from build123d import *

# Parameters (mm, degrees)
SKETCH1_R           = 2.286
BOSS_EXTRUDE1_DEPTH = 1.5875
SKETCH2_R           = 2.286
CUT_EXTRUDE1_DEPTH  = 118.348360795
SKETCH3_R           = 1.27
CUT_EXTRUDE2_DEPTH  = 118.348360795
SKETCH4_W           = 2.54
SKETCH4_H           = 6.9596
BOSS_EXTRUDE2_DEPTH = 8.89
CHAMFER1_SIZE       = 1.27
SKETCH5_W           = 10.16
SKETCH5_H           = 2.54
CUT_EXTRUDE3_DEPTH  = 118.673912678
SKETCH6_R           = 1.27
CUT_EXTRUDE4_DEPTH  = 8.89


with BuildPart() as part:
    # Sketch1 → Boss-Extrude1 (new body)
    with BuildSketch(Plane(origin=(0, 0, 0), x_dir=(1, 0, 0), z_dir=(0, 1, 0))):
        Polygon((-25.4, 86.995), (-63.43142, 86.995), (-63.43142, 60.96), (-78.74, 60.96), (-78.74, 25.4), (-71.12, 25.4), (-71.12, -25.4), (-78.74, -25.4), (-78.74, -60.96), (-63.43142, -60.96), (-63.43142, -86.995), (-25.4, -86.995), (-25.4, -79.375), (25.4, -79.375), (25.4, -86.995), (63.43142, -86.995), (63.43142, -60.96), (78.74, -60.96), (78.74, -25.4), (71.12, -25.4), (71.12, 25.4), (78.74, 25.4), (78.74, 60.96), (63.43142, 60.96), (63.43142, 86.995), (25.4, 86.995), (25.4, 79.375), (-25.4, 79.375), align=None)
        with Locations(Location((-57.15, 76.2, 0), (0, 0, 270))):
            Circle(SKETCH1_R, mode=Mode.SUBTRACT)
        with Locations(Location((57.15, 76.2, 0), (0, 0, 270))):
            Circle(SKETCH1_R, mode=Mode.SUBTRACT)
        with Locations(Location((57.15, -76.2, 0), (0, 0, 270))):
            Circle(SKETCH1_R, mode=Mode.SUBTRACT)
        with Locations(Location((-57.15, -76.2, 0), (0, 0, 270))):
            Circle(SKETCH1_R, mode=Mode.SUBTRACT)
    extrude(amount=BOSS_EXTRUDE1_DEPTH)

    # Sketch2 → Cut-Extrude1 (cut, through all)
    with BuildSketch(Plane(origin=(0, 1.5875, 0), x_dir=(1, 0, 0), z_dir=(0, 1, 0))):
        with Locations(Location((-73.66, -30.48, 0), (0, 0, 270))):
            Circle(SKETCH2_R)
        with Locations(Location((-73.66, -55.88, 0), (0, 0, 270))):
            Circle(SKETCH2_R)
        with Locations(Location((73.66, -55.88, 0), (0, 0, 90))):
            Circle(SKETCH2_R)
        with Locations(Location((73.66, -30.48, 0), (0, 0, 90))):
            Circle(SKETCH2_R)
        with Locations(Location((73.66, 30.48, 0), (0, 0, 270))):
            Circle(SKETCH2_R)
        with Locations(Location((73.66, 55.88, 0), (0, 0, 270))):
            Circle(SKETCH2_R)
        with Locations(Location((-73.66, 55.88, 0), (0, 0, 90))):
            Circle(SKETCH2_R)
        with Locations(Location((-73.66, 30.48, 0), (0, 0, 90))):
            Circle(SKETCH2_R)
    extrude(amount=-CUT_EXTRUDE1_DEPTH, mode=Mode.SUBTRACT)

    # Sketch3 → Cut-Extrude2 (cut, through all)
    with BuildSketch(Plane(origin=(0, 1.5875, 0), x_dir=(1, 0, 0), z_dir=(0, 1, 0))):
        with Locations(Location((-50.73142, 66.675, 0), (0, 0, 270))):
            Circle(SKETCH3_R)
        with Locations(Location((10.99058, 66.675, 0), (0, 0, 270))):
            Circle(SKETCH3_R)
        with Locations(Location((10.99058, 12.065, 0), (0, 0, 270))):
            Circle(SKETCH3_R)
        with Locations(Location((-50.73142, 12.065, 0), (0, 0, 270))):
            Circle(SKETCH3_R)
    extrude(amount=-CUT_EXTRUDE2_DEPTH, mode=Mode.SUBTRACT)

    # Sketch4 → Boss-Extrude2 (add)
    with BuildSketch(Plane(origin=(0, 1.5875, 0), x_dir=(1, 0, 0), z_dir=(0, 1, 0))):
        Polygon((-15.748, -44.4754), (55.88, -44.4754), (58.42, -44.4754), (58.42, -41.9354), (-18.288, -41.9354), (-18.288, -44.4754), align=None)
        with Locations((-17.018, -54.3052)):
            Rectangle(SKETCH4_W, SKETCH4_H)
        Polygon((-15.748, -64.135), (55.88, -64.135), (58.42, -64.135), (58.42, -66.675), (-18.288, -66.675), (-18.288, -64.135), align=None)
        with Locations((57.15, -54.3052)):
            Rectangle(SKETCH4_W, SKETCH4_H)
    extrude(amount=BOSS_EXTRUDE2_DEPTH)

    # Chamfer1
    chamfer1_edges = [part.edges().sort_by_distance(p)[0] for p in [
        (20.066, 10.4775, 44.4754),
        (58.42, 10.4775, 43.2054),
        (20.066, 10.4775, 41.9354),
        (-18.288, 10.4775, 43.2054),
        (20.066, 10.4775, 64.135),
        (-18.288, 10.4775, 65.405),
        (20.066, 10.4775, 66.675),
        (58.42, 10.4775, 65.405),
        (-17.018, 10.4775, 50.8254),
        (-18.288, 10.4775, 54.3052),
        (-17.018, 10.4775, 57.785),
        (-15.748, 10.4775, 54.3052),
        (58.42, 10.4775, 54.3052),
        (57.15, 10.4775, 50.8254),
        (55.88, 10.4775, 54.3052),
        (57.15, 10.4775, 57.785),
    ]]
    chamfer(chamfer1_edges, length=CHAMFER1_SIZE - 0.0001)  # a hair under: the kernel refuses the full size

    # Sketch5 → Cut-Extrude3 (cut, through all)
    with BuildSketch(Plane(origin=(0, 1.5875, 0), x_dir=(1, 0, 0), z_dir=(0, 1, 0))):
        with Locations((-6.858, -40.6654)):
            Rectangle(SKETCH5_W, SKETCH5_H)
        with Locations((46.99, -40.6654)):
            Rectangle(SKETCH5_W, SKETCH5_H)
        with Locations((46.99, -67.945)):
            Rectangle(SKETCH5_W, SKETCH5_H)
        with Locations((-6.858, -67.945)):
            Rectangle(SKETCH5_W, SKETCH5_H)
    extrude(amount=-CUT_EXTRUDE3_DEPTH, mode=Mode.SUBTRACT)

    # Sketch6 → Cut-Extrude4 (cut)
    with BuildSketch(Plane(origin=(0, 1.5875, 0), x_dir=(1, 0, 0), z_dir=(0, 1, 0))):
        with Locations(Location((-33.02, -29.21, 0), (0, 0, 270))):
            Circle(SKETCH6_R)
        with Locations(Location((-33.02, -45.72, 0), (0, 0, 270))):
            Circle(SKETCH6_R)
    extrude(amount=-CUT_EXTRUDE4_DEPTH, mode=Mode.SUBTRACT)


solid = part.part
Input: part model. Units: mm. Frame: model coordinates. A direction names the side the tool comes from. Give positions to 0.01 mm unless a question says otherwise; leave off trailing zeros. Loops run counter-clockwise (first coordinate to the right, second up) from the corner with the lowest first, then second, coordinate; pieces in that order, holes last. Notation, with made-up numbers: (-39, 58.5) -> (-20, 58.5) arc R29 cw to (-20, 80.5) -> close; hole circle Ø6 at (21, 7.25). An arc over 180 degrees is marked (long way). Answer as a JSON object with one key per item and string values. Group by question number.
Item 1: Cut plane B-B, the plane z = -55.88. Return the cut outline in (x, y), and give its area (3 significant figures).
Item 2: Line query: probe 1 along X at (y, z) = (0.95, -55.88); probe 2 along Z at (x, y) = (33.5, 8) (3 decimals); probe 3 along X at (y, z) = (1.5, -18.5). Output: solid intervals per line, ascending.
Item 3: Reachability of faces 3 (the flat face through (-15.748, 5, 54)), 4 (the flat face through (58.42, 5, 54)), 5 (the flat face through (20, 5, 44.475)) from +Z, -Z, +X, -X, +Y, -Y: full face, straight path, thin tool, end or side. Return the list, or none.
Item 4: Pull-direction query (Z, two-part tool) for faces 1 (the flat face through (-18.288, 5, 54)), 2 (the cylindrical face through (-75.69, 0.8, 56.93)); classes: released by +Z, released by -Z, zero draft, split by the parting line, or undercut.
Item 5: Cut plane C-C, the plane y = 7.25. Return the cut outline in (x, z) (3 decimals).
Item 6: Cut plane D-D, the plane x = -57.15. Return the cut outline in (y, z) (1 decimal).
Item 7: Cut plane A-A, the plane x = -73.66. Return the cut outline in (y, z), and give its area (3 significant figures).
Item 8: Pin query (flat end, axial travel): P1, Ø0.8, axis at x = -68.5, y = 1, coming from the -Z side; P2, Ø4, axis at x = 57.15, z = -76.2, coming from the +Y side; P3, Ø3, axis at x = 27.5, y = 5.5, coming from the -Z side; P4, Ø3, axis at x = -43, z = -22, coming from the +Y side. Return the tip coordinate at first contact, or that it passes through.
Checks:
{
 "1": {"outline": "(-78.74, 0) -> (-75.95, 0) -> (-75.95, 1.59) -> (-78.74, 1.59) -> close; (-71.37, 0) -> (71.37, 0) -> (71.37, 1.59) -> (-71.37, 1.59) -> close; (75.95, 0) -> (78.74, 0) -> (78.74, 1.59) -> (75.95, 1.59) -> close", "area": "235 mm²"},
 "2": {"probe 1": "x = -78.74 to -75.95, -71.37 to 71.37, 75.95 to 78.74", "probe 2": "z = 41.935 to 44.475, 64.135 to 66.675", "probe 3": "x = -71.12 to 71.12"},
 "3": {"face 3": "+Y", "face 4": "+Z, -Z, +X, +Y", "face 5": "+X, -X, +Y"},
 "4": {"face 1": "zero draft", "face 2": "undercut"},
 "5": {"outline": "(-18.288, 41.935) -> (58.42, 41.935) -> (58.42, 44.475) -> (-18.288, 44.475) -> close; (-18.288, 50.825) -> (-15.748, 50.825) -> (-15.748, 57.785) -> (-18.288, 57.785) -> close; (-18.288, 64.135) -> (58.42, 64.135) -> (58.42, 66.675) -> (-18.288, 66.675) -> close; (55.88, 50.825) -> (58.42, 50.825) -> (58.42, 57.785) -> (55.88, 57.785) -> close"},
 "6": {"outline": "(0, -87) -> (1.6, -87) -> (1.6, -78.5) -> (0, -78.5) -> close; (0, -73.9) -> (1.6, -73.9) -> (1.6, 73.9) -> (0, 73.9) -> close; (0, 78.5) -> (1.6, 78.5) -> (1.6, 87) -> (0, 87) -> close"},
 "7": {"outline": "(0, -60.96) -> (1.59, -60.96) -> (1.59, -58.17) -> (0, -58.17) -> close; (0, -53.59) -> (1.59, -53.59) -> (1.59, -32.77) -> (0, -32.77) -> close; (0, -28.19) -> (1.59, -28.19) -> (1.59, -25.4) -> (0, -25.4) -> close; (0, 25.4) -> (1.59, 25.4) -> (1.59, 28.19) -> (0, 28.19) -> close; (0, 32.77) -> (1.59, 32.77) -> (1.59, 53.59) -> (0, 53.59) -> close; (0, 58.17) -> (1.59, 58.17) -> (1.59, 60.96) -> (0, 60.96) -> close", "area": "83.9 mm²"},
 "8": {"P1": "stops at z = -60.96", "P2": "passes through", "P3": "stops at z = 41.94", "P4": "stops at y = 1.59"}
}
